Part model, mm, in its own coordinate system. A direction names the side the tool comes from. Give positions to 0.01 mm unless a question says otherwise; leave off trailing zeros. Order: outer loops, then holes, each group sorted by start corner. A loop starts at its lowest first (then second) coordinate and runs counter-clockwise, first axis right, second up. Notation, with made-up numbers: (88, -6.75) -> (138, -6.75) arc R26 ccw to (138, 29.25) -> close; hole circle Ø1 at (4.5, 35.25). An arc over 180 degrees is marked (long way). Write item = value, one per line. Start each with the question number.
(1) Flat gauge pins, fed straight in: pin 1 (6 mm diameter, centred on x = -18.5, z = 49.5, fed in from -Y); pin 2 (7.5 mm diameter, centred on y = -9, z = 32.5, fed in from -X); pin 3 (11 mm diameter, centred on x = -15, z = 30, fed in from +Y); pin 4 (2 mm diameter, centred on y = 22, z = 78.5, fed in from +X). Where does each tip first touch, or does it go through?
(2) Saw through at C-C, the plane y = 30. List the corners of the cut face in (x, z), then the cut area to 3 significant figures.
(3) Saw through at A-A, the plane z = 70. List the corners of the cut face in (x, y).
(4) Saw through at D-D, the plane x = -3.5. List the corners of the cut face in (y, z), then the cut area to 3 significant figures.
(5) Saw through at B-B, the plane x = -17.5. List the corners of the cut face in (y, z).
(6) Two-plate mould, pull along Y, no slides. Class faces 1 (the flat face through (-15.07, -18.521, 32.605)), 2 (the flat face through (-12, -20, 53)), 3 (the flat face through (-13, -17, 36)): pulls with the +Y half, pulls with the -Y half, needs draft (parallel to the pull), parting line crosses it, or undercut.
(7) Which spindle directions (+Z, -Z, +X, -X, +Y, -Y) get a long thin tool onto all of the face, cutting with end or side? Do faces 4 (the flat face through (-15.07, 18.521, 32.605)), 5 (the flat face through (-10, 0, 27)), 6 (the flat face through (-20, -5, 65)), 7 (the flat face through (-5, 0, 50)). Say none if no direction does.
(8) Probe line 1 along Y through (x, z) = (-30, 8); line 2 along Z through (x, y) = (-18, -0.5); line 3 along Z through (x, y) = (-12.75, 0). List the from-to ranges inside material, lowest first. Write a range as from..to.
from build123d import *

# Parameters (mm, degrees)
SKETCH1_W                      = 80
SKETCH1_H                      = 80
BOSS_EXTRUDE1_DEPTH            = 10
SKETCH2_W                      = 40
SKETCH2_H                      = 40
BOSS_EXTRUDE2_DEPTH            = 80
F_4_0_4_DIAMETER_HOLE1_D       = 4
CUT_EXTRUDE1_REACH             = 117.326
CUT_EXTRUDE1_DIRECTION_2_REACH = 117.326
CUT_EXTRUDE2_REACH             = 117.326
SKETCH10_W                     = 10
SKETCH10_H                     = 30
BOSS_EXTRUDE3_DEPTH            = 3
F_12_0_MM_DOWEL_HOLES1_D       = 12
CHAMFER1_SIZE                  = 5


with BuildPart() as part:
    # Sketch1 → Boss-Extrude1 (new body)
    with BuildSketch(Plane(origin=(0, 0, 0), x_dir=(0, 1, 0), z_dir=(0, 0, 1))):
        Rectangle(SKETCH1_W, SKETCH1_H)
    extrude(amount=BOSS_EXTRUDE1_DEPTH)

    # Sketch2 → Boss-Extrude2 (add)
    with BuildSketch(Plane.XY.offset(10)):
        Rectangle(SKETCH2_W, SKETCH2_H)
    extrude(amount=BOSS_EXTRUDE2_DEPTH)

    # Ø4.0 (4) Diameter Hole1 (through all)
    with Locations(Plane.XY.offset(10)):
        with Locations((-30, -30), (30, -30)):
            f_4_0_4_diameter_hole1 = Hole(F_4_0_4_DIAMETER_HOLE1_D / 2)

    # Sketch9 → Cut-Extrude1 (cut, up to next)
    with BuildSketch(Plane.XZ.offset(20), mode=Mode.PRIVATE) as cut_extrude1_sk1:
        Polygon((-10, 90), (40, 90), (40, 45), (40, 0), (0, 0), (0, 50), (-10, 50), align=None)
    cut_extrude1_tool1 = extrude(cut_extrude1_sk1.sketch, amount=-CUT_EXTRUDE1_REACH, mode=Mode.PRIVATE) & part.part
    add(cut_extrude1_tool1.solids().sort_by_distance((17.5, -20, 47.5))[0], mode=Mode.SUBTRACT)

    # Sketch9 → Cut-Extrude1 direction 2 (cut, up to next)
    with BuildSketch(Plane.XZ.offset(20), mode=Mode.PRIVATE) as cut_extrude1_direction_2_sk1:
        Polygon((-10, 90), (40, 90), (40, 45), (40, 0), (0, 0), (0, 50), (-10, 50), align=None)
    cut_extrude1_direction_2_tool1 = extrude(cut_extrude1_direction_2_sk1.sketch, amount=CUT_EXTRUDE1_DIRECTION_2_REACH, mode=Mode.PRIVATE) & part.part
    add(cut_extrude1_direction_2_tool1.solids().sort_by_distance((17.5, -20, 47.5))[0], mode=Mode.SUBTRACT)

    # Sketch10 → Cut-Extrude2 (cut, up to next)
    with BuildSketch(Plane.XZ.offset(20), mode=Mode.PRIVATE) as cut_extrude2_sk1:
        with Locations((-15, 25)):
            Rectangle(SKETCH10_W, SKETCH10_H)
    cut_extrude2_tool1 = extrude(cut_extrude2_sk1.sketch, amount=-CUT_EXTRUDE2_REACH, mode=Mode.PRIVATE) & part.part
    add(cut_extrude2_tool1.solids().sort_by_distance((-15, -20, 25))[0], mode=Mode.SUBTRACT)

    # Sketch11 → Boss-Extrude3 (add)
    with BuildSketch(Plane.XZ.offset(20)):
        Polygon((-20, 40), (-10, 25), (-10, 40), align=None)
    boss_extrude3 = extrude(amount=-BOSS_EXTRUDE3_DEPTH)

    # Mirror2: Boss-Extrude3 across plane
    add(boss_extrude3.mirror(Plane.ZX))

    # Sketch13 → Ø4.0 (4) Diameter Hole2 (revolve, cut)
    with BuildSketch(Plane(origin=(-10, 10, 25), x_dir=(0, 0, 1), z_dir=(0, 1, 0))):
        Polygon((0, 0), (0, 11.301721238), (2, 10.1), (2, 0), align=None)
    f_4_0_4_diameter_hole2 = revolve(axis=Axis((-16.35, 10, 25), (1, 0, 0)), mode=Mode.SUBTRACT)

    # Ø12.0 mm Dowel Holes1 (through all)
    with Locations(Plane(origin=(-20, 0, 0), x_dir=(0, -1, 0), z_dir=(-1, 0, 0))):
        with Locations((0, 70)):
            Hole(F_12_0_MM_DOWEL_HOLES1_D / 2)

    # Chamfer1
    chamfer1_edges = [part.edges().sort_by_distance(p)[0] for p in [
        (-5, 20, 10),
        (-5, -20, 10),
        (-10, 0, 10),
    ]]
    chamfer(chamfer1_edges, length=CHAMFER1_SIZE)

    # Mirror3: Ø4.0 (4) Diameter Hole1, Ø4.0 (4) Diameter Hole2 across plane
    add(f_4_0_4_diameter_hole1.mirror(Plane.ZX), mode=Mode.SUBTRACT)
    add(f_4_0_4_diameter_hole2.mirror(Plane.ZX), mode=Mode.SUBTRACT)


solid = part.part
Results list:
q1.pin_1 = -20
q1.pin_2 = -10
q1.pin_3 = 20
q1.pin_4 = through
q2.outline = (-40, 0) -> (-32, 0) -> (-32, 10) -> (-40, 10) -> close; (-28, 0) -> (0, 0) -> (0, 10) -> (-28, 10) -> close
q2.area = 360 mm^2
q3.outline = (-20, -20) -> (-10, -20) -> (-10, -6) -> (-20, -6) -> close; (-20, 6) -> (-10, 6) -> (-10, 20) -> (-20, 20) -> close
q4.outline = (-40, 0) -> (40, 0) -> (40, 10) -> (25, 10) -> (20, 15) -> (20, 50) -> (-20, 50) -> (-20, 15) -> (-25, 10) -> (-40, 10) -> close; hole circle Ø4 at (-10, 25); hole circle Ø4 at (10, 25)
q4.area = 2,400 mm^2
q5.outline = (-40, 0) -> (40, 0) -> (40, 10) -> (-40, 10) -> close; (-20, 36.25) -> (-17, 36.25) -> (-17, 40) -> (17, 40) -> (17, 36.25) -> (20, 36.25) -> (20, 90) -> (-20, 90) -> close; hole circle Ø12 at (0, 70)
q6.face_1 = needs draft
q6.face_2 = pulls with the -Y half
q6.face_3 = undercut
q7.face_4 = -X, +Y, -Y
q7.face_5 = -X
q7.face_6 = +Z, -X, +Y, -Y
q7.face_7 = +Z, +X, +Y, -Y
q8.line_1 = -40..-32, -28..28, 32..40
q8.line_2 = 0..10, 40..64.02, 75.98..90
q8.line_3 = 0..12.25, 40..64, 76..90
